For this review, use the dimensioned drawing (mm, ordinates from the lowest corner) and the shaded views. Give positions to 0.01 mm unless a question says otherwise; leave off trailing zeros. Order: outer loops, then holes, each group sorted by start corner. A loop starts at its lowest first (then second) coordinate and runs counter-clockwise, first axis right, second up. Notation, with made-up numbers: (18.25, 67.5) - (44.25, 67.5) arc R20 ccw to (44.25, 88.5) - close; hole circle Ø7 at (67.5, 79.25). An arc over 180 degrees is marked (long way). Use a Markdown table: item, result. Add a question column.
1) Wall thickness on L1, parallel to X at y = 0.7, z = 50; L2, parallel to X at y = 2.55, z = 28.5; L3, parallel to Z at x = 33, y = 1.15: over which ranges is each line inside the solid? List them lowest first.
2) Clearance check with flat-ended pins moving along their axes: P1, Ø2.5, axis at x = 65, z = 5, coming from the +Y side; P2, Ø5, axis at x = 35, z = 6, coming from the +Y side. State where each tip first meets the part, or that it passes through.
3) We need section A-A on z = 46.5. Write out the cut boundary in (x, y), then the cut area to 3 significant figures.
4) We need section B-B on x = 40. Write out the cut boundary in (y, z), then the cut area to 3 significant figures.
5) We need section C-C on x = 50. Write out the cut boundary in (y, z).
6) We need section D-D on x = 16.5. Write out the cut boundary in (y, z).
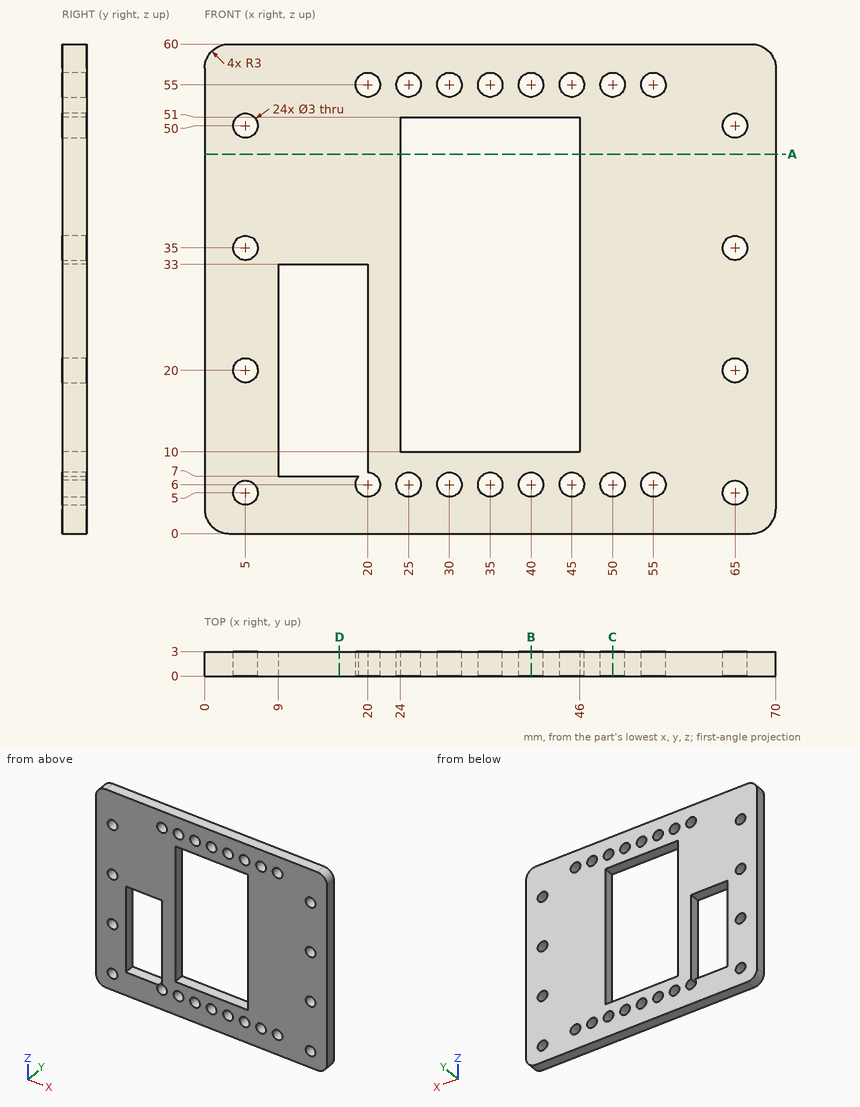
Checked values:
| question | item | result |
|---|---|---|
| 1 | L1 | 0 to 3.5, 6.5 to 24, 46 to 63.5, 66.5 to 70 |
| 1 | L2 | 0 to 9, 20 to 24, 46 to 70 |
| 1 | L3 | 0 to 10, 51 to 60 |
| 2 | P1 | through |
| 2 | P2 | y = 3 |
| 3 | outline | (0, 0) - (24, 0) - (24, 3) - (0, 3) - close; (46, 0) - (70, 0) - (70, 3) - (46, 3) - close |
| 3 | area | 144 mm² |
| 4 | outline | (0, 0) - (3, 0) - (3, 4.5) - (0, 4.5) - close; (0, 7.5) - (3, 7.5) - (3, 10) - (0, 10) - close; (0, 51) - (3, 51) - (3, 53.5) - (0, 53.5) - close; (0, 56.5) - (3, 56.5) - (3, 60) - (0, 60) - close |
| 4 | area | 39.0 mm² |
| 5 | outline | (0, 0) - (3, 0) - (3, 4.5) - (0, 4.5) - close; (0, 7.5) - (3, 7.5) - (3, 53.5) - (0, 53.5) - close; (0, 56.5) - (3, 56.5) - (3, 60) - (0, 60) - close |
| 6 | outline | (0, 0) - (3, 0) - (3, 7) - (0, 7) - close; (0, 33) - (3, 33) - (3, 60) - (0, 60) - close |
